Input: dimensioned drawing with shaded views. Units: mm. Origin: part minimum x, y, z. Give positions to 0.01 mm unless a question says otherwise; leave off trailing zeros. Write each loop counter-clockwise with the first axis right and the second up, starting at its lowest first coordinate (ties: lowest second). Pieces come first, ordered by that corner, then holes. Notation, with made-up numbers: (89, 2) - (120, 2) arc R7 ccw to (120, 14) - close; hole circle Ø10 at (41, 57). An arc over 180 degrees is marked (long way). Answer as CSV lines item,"result".
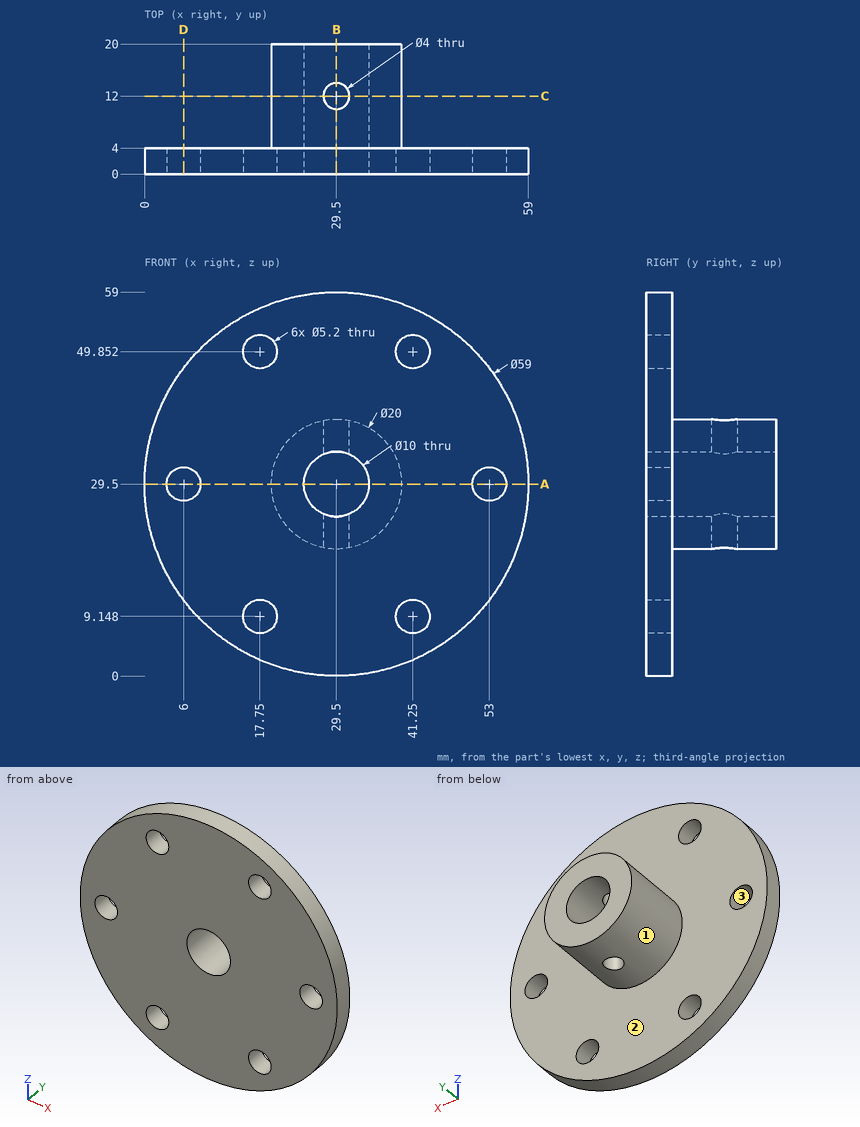
Item 1: Contact query for flat-ended pins moving along their axis: pin 1 (11.5 mm diameter, centred on x = 29.5, z = 29.5, fed in from -Y); pin 2 (10 mm diameter, centred on x = 10, z = 11.5, fed in from +Y); pin 3 (12 mm diameter, centred on y = 6.5, z = 17, fed in from -X); pin 4 (1 mm diameter, centred on y = 5.5, z = 28, fed in from +X). Output: stop coordinate, or through.
The answers:
pin 1,"y = 0"
pin 2,"y = 4"
pin 3,"x = 0.85"
pin 4,"x = 39.45"
Item 2: Ray query, line 1 (Y direction, x = 29.5, z = 36.85); line 2 (X direction, y = 0.8, z = 29.5); line 3 (Z direction, x = 42.5, y = 2). Return the intervals inside material, ascending. Write a range as from..to.
The answers:
line 1,"0..10, 14..20"
line 2,"0..3.4, 8.6..24.5, 34.5..50.4, 55.6..59"
line 3,"3.02..6.87, 11.43..47.57, 52.13..55.98"
Item 3: Cut plane C-C on y = 12. Return the cut outline in (x, z).
The answers:
outline,"(27.5, 19.7) - (27.5, 24.92) arc R5 cw to (27.5, 34.08) - (27.5, 39.3) arc R10 ccw to start; (31.5, 19.7) arc R10 ccw to (31.5, 39.3) - (31.5, 34.08) arc R5 cw to (31.5, 24.92) - close"
Item 4: Mould query, pull axis X, two halves, no side actions, for the marked faces 1, 2 and 3. Classes: +X half, -X half, draft (parallel to the pull), parting line (faces both ways), or undercut.
The answers:
face 1,"parting line"
face 2,"draft"
face 3,"undercut"
Item 5: Cut plane A-A on z = 29.5. Return the cut outline in (x, y).
The answers:
outline,"(0, 0) - (3.4, 0) - (3.4, 4) - (0, 4) - close; (8.6, 0) - (24.5, 0) - (24.5, 20) - (19.5, 20) - (19.5, 4) - (8.6, 4) - close; (34.5, 0) - (50.4, 0) - (50.4, 4) - (39.5, 4) - (39.5, 20) - (34.5, 20) - close; (55.6, 0) - (59, 0) - (59, 4) - (55.6, 4) - close"
Item 6: Cut plane D-D on x = 6. Return the cut outline in (y, z).
The answers:
outline,"(0, 11.67) - (4, 11.67) - (4, 26.9) - (0, 26.9) - close; (0, 32.1) - (4, 32.1) - (4, 47.33) - (0, 47.33) - close"
Item 7: Cut plane B-B on x = 29.5. Return the cut outline in (y, z), plus the area to 3 significant figures.
The answers:
outline,"(0, 0) - (4, 0) - (4, 19.5) - (10, 19.5) - (10, 24.5) - (0, 24.5) - close; (0, 34.5) - (10, 34.5) - (10, 39.5) - (4, 39.5) - (4, 59) - (0, 59) - close; (14, 19.5) - (20, 19.5) - (20, 24.5) - (14, 24.5) - close; (14, 34.5) - (20, 34.5) - (20, 39.5) - (14, 39.5) - close"
area,"316 mm²"
